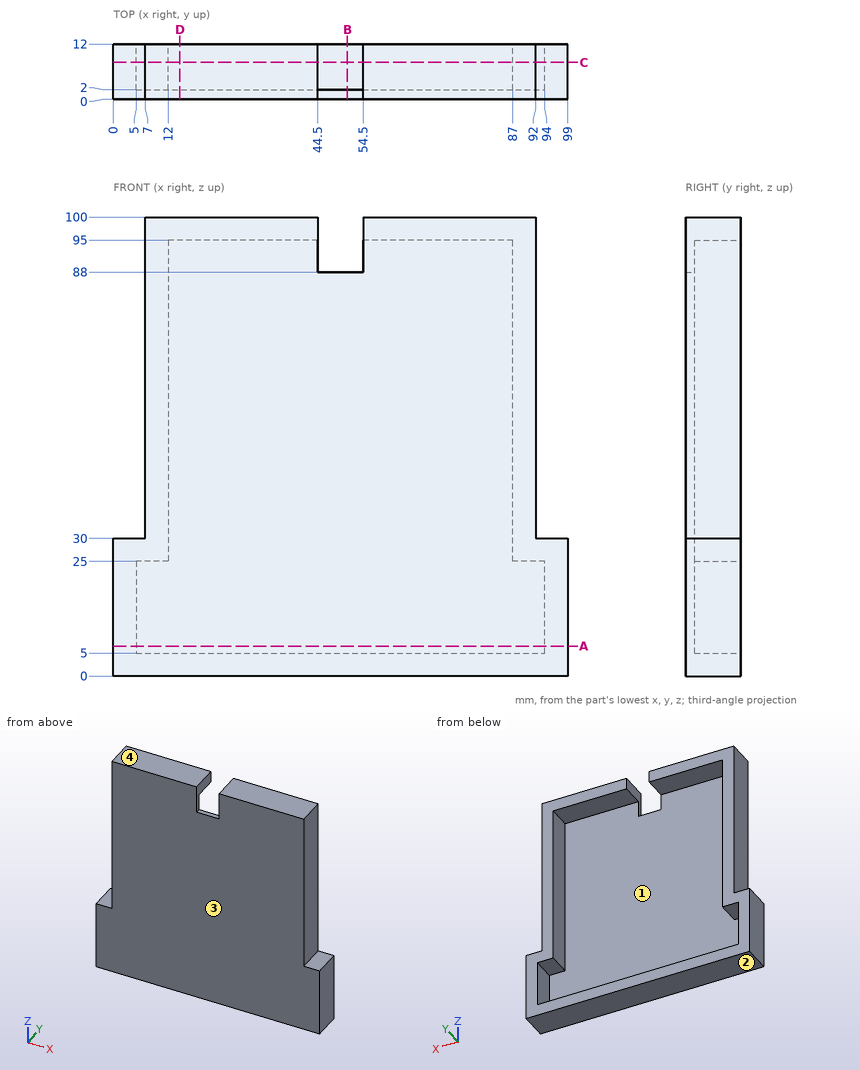
Here's the drawing with two shaded views (mm, measured from the low corner). I have some questions. Give positions to 0.01 mm unless a question says otherwise; leave off trailing zeros. Loops run counter-clockwise (first coordinate to the right, second up) from the corner with the lowest first, then second, coordinate; pieces in that order, holes last. Notation, with made-up numbers: (88.5, 55.25) -> (106.5, 55.25) arc R16 cw to (106.5, 62.25) -> close; hole circle Ø3 at (63.25, -37). An arc over 180 degrees is marked (long way). Answer as a JSON object with one key per item and string values. Group by question number.
Item 1: I need wall thicknesses on L1, parallel to X at y = 11.5, z = 14.5; L2, parallel to X at y = 3.25, z = 85; L3, parallel to Z at x = 84, y = 10.5. Which ranges of each line are inside material? Lowest first, please.
Item 2: Will these pins go through, and if not, where does the flat tip stop? pin 1 (1.5 mm diameter, centred on x = 21.5, z = 22.5, fed in from +Y); pin 2 (1.5 mm diameter, centred on x = 35, z = 79, fed in from -Y); pin 3 (1 mm diameter, centred on y = 8, z = 89.5, fed in from -X); pin 4 (3.5 mm diameter, centred on x = 2.5, y = 7.5, fed in from +Z).
Item 3: Imagine slicing it at B-B on x = 51. Write out the boundary of the cut face in (y, z).
Item 4: Imagine slicing it at A-A on z = 6.5. Write out the boundary of the cut face in (x, y), then the cut area to 3 significant figures.
Item 5: Imagine slicing it at C-C on y = 8. Write out the boundary of the cut face in (x, z), then the cut area to 3 significant figures.
Item 6: Imagine slicing it at D-D on x = 14.5. Write out the boundary of the cut face in (y, z), then the cut area to 3 significant figures.
Item 7: Thinking about a two-plate mould opening in Z: for the marked faces 1, 2, 3 and 4, which applies, pulls with the +Z half, pulls with the -Z half, needs draft (parallel to the pull), parting line crosses it, or undercut?
Answer list:
{
 "1": {"L1": "x = 0 to 5, 94 to 99", "L2": "x = 7 to 12, 87 to 92", "L3": "z = 0 to 5, 95 to 100"},
 "2": {"pin 1": "stops at y = 2", "pin 2": "stops at y = 0", "pin 3": "stops at x = 7", "pin 4": "stops at z = 30"},
 "3": {"outline": "(0, 0) -> (12, 0) -> (12, 5) -> (2, 5) -> (2, 88) -> (0, 88) -> close"},
 "4": {"outline": "(0, 0) -> (99, 0) -> (99, 12) -> (94, 12) -> (94, 2) -> (5, 2) -> (5, 12) -> (0, 12) -> close", "area": "298 mm2"},
 "5": {"outline": "(0, 0) -> (99, 0) -> (99, 30) -> (92, 30) -> (92, 100) -> (54.5, 100) -> (54.5, 95) -> (87, 95) -> (87, 25) -> (94, 25) -> (94, 5) -> (5, 5) -> (5, 25) -> (12, 25) -> (12, 95) -> (44.5, 95) -> (44.5, 100) -> (7, 100) -> (7, 30) -> (0, 30) -> close", "area": "1,840 mm2"},
 "6": {"outline": "(0, 0) -> (12, 0) -> (12, 5) -> (2, 5) -> (2, 95) -> (12, 95) -> (12, 100) -> (0, 100) -> close", "area": "300 mm2"},
 "7": {"face 1": "undercut", "face 2": "pulls with the -Z half", "face 3": "needs draft", "face 4": "pulls with the +Z half"}
}
